CAD build for the part. Positions are in the model's coordinates, mm. A direction names the side the tool comes from. Coordinates: 2 decimals unless noted, no trailing zeros. Loops run counter-clockwise (first coordinate to the right, second up) from the corner with the lowest first, then second, coordinate; pieces in that order, holes last.
1) Wall check: line 1 along Z through (x, y) = (-1.5, 65.75); line 2 along Y through (x, z) = (0.25, 3); line 3 along X through (y, z) = (57.25, 3.25). Give the ranges that are in metal, low to high.
2) Pin check, flat tips, straight feed: pin 1 Ø2 at (x, z) = (7.5, 3.5) entering from -Y; pin 2 Ø4 at (x, z) = (5, 7) entering from -Y; pin 3 Ø10 at (x, y) = (-1.5, 49.5) entering from +Z. Stop position of each tip, or through.
3) Which spindle directions (+Z, -Z, +X, -X, +Y, -Y) get a long thin tool onto all of the face, cutting with end or side? Do faces 1 (the flat face through (0, 57, 0)), 2 (the flat face through (2.9, 49.6, 7)). Say none if no direction does.
4) Saw through at A-A, the plane x = 0. Write the cut outline in (y, z).
5) Saw through at C-C, the plane z = 6.75. Write the cut outline in (x, y), and give its area (3 significant figures).
6) Saw through at B-B, the plane y = 57. Write the cut outline in (x, z).
Autodesk Inventor part; units mm, degrees
ref_plane "YZ Plane" through (0, 0, 0) normal (1, 0, 0) x (0, 1, 0)
ref_plane "XZ Plane" through (0, 0, 0) normal (0, 1, 0) x (-1, 0, 0)
ref_plane "XY Plane" through (0, 0, 0) normal (0, 0, 1) x (1, 0, 0)
sketch "Sketch1" plane through (0, 0, 0) normal (0, 0, 1) x (1, 0, 0)
  line L0 (14, 0) -> (-14, 0)
  line L1 (0, 0) -> (0, 47)
  line L2 (0, 47) -> (0, 57)
  circle A0 centre (0, 57) radius 10
  circle A1 centre (0, 57) radius 8.5
  dimension "d0" = 47
  dimension "d1" = 10
  dimension "d2" = 1.5
extrude "Extrusion1" add sketch "Sketch1" along normal blind 7
sketch "Sketch2" plane through (0, 57, 0) normal (0, 0, -1) x (-1, 0, 0)
  circle A0 centre (0, 0) radius 7.75
  point P0 (0, -57)
  dimension "d5" = 15.5
extrude "Extrusion2" add sketch "Sketch2" against normal up to surface (7 mm away)
sketch "Sketch3" plane through (0, 57, 0) normal (0, 0, -1) x (-1, 0, 0)
  circle A0 centre (0, 0) radius 7.75
  circle A1 centre (0, 0) radius 10
  point P0 (0, -57)
extrude "Extrusion3" add sketch "Sketch3" against normal blind 4 contours A0 | A1
sketch "Sketch4" plane through (0, 0, 0) normal (1, 0, 0) x (0, 1, 0)
  line L0 (57, 0) -> (57, 7)
  line L1 (48.5, 7) -> (65.5, 7)
  line L2 (57, 7) -> (57, 10)
  line L3 (64.75, 4) -> (64.75, 7)
  line L4 (49.25, 4) -> (49.25, 7)
  arc A0 (64.75, 7) -> (49.25, 7) centre (57, -1.5104) ccw
  point P0 (0, 0)
  dimension "d10" = 3
revolve "Revolution1" add sketch "Sketch4" angle 360 about axis through (0, 57, 7) along (0, 0, 1) picked at (52.6027, 7.5441) contours A0 L2 L1
sketch "Sketch5" plane through (0, 57, 7) normal (0, 0, 1) x (1, 0, 0)
  circle A0 centre (0, 0) radius 7.75
  circle A1 centre (0, 0) radius 8.5
  point P0 (0, -57)
extrude "Extrusion4" add sketch "Sketch5" against normal up to surface (7 mm away)
properties part number "Button1"
Data:
1. line 1: z = 0 to 7
1. line 2: y = 47 to 67
1. line 3: x = -10 to 10
2. pin 1: stops at y = 49.4
2. pin 2: stops at y = 47.46
2. pin 3: stops at z = 9.69
3. face 1: -Z, +X, -X, +Y, -Y
3. face 2: +Z
4. outline: (47, 0) - (67, 0) - (67, 7) - (64.75, 7) arc R11.51 ccw to (49.25, 7) - (47, 7) - close
5. outline: circle Ø20 at (0, 57)
5. area: 314 mm2
6. outline: (-10, 0) - (10, 0) - (10, 7) - (7.75, 7) arc R11.51 ccw to (-7.75, 7) - (-10, 7) - close
